The model under review builds one solid part; all positions refer to its coordinate system, in mm. Face numbers are marked on the shaded views. A direction names the side the tool comes from. Round coordinates to 2 decimals unless told otherwise and drop trailing zeros. Write each loop counter-clockwise with the first axis right and the second up, starting at its lowest first coordinate (ties: lowest second). Pieces come first, ordered by that corner, then holes. Notation, with made-up numbers: (28, -16.5) - (84, -16.5) arc R16 ccw to (84, 14.5) - close; hole circle Ø2 at (75, 54). An arc over 180 degrees is marked (long way). Return JSON: item names as keys, results as strings.
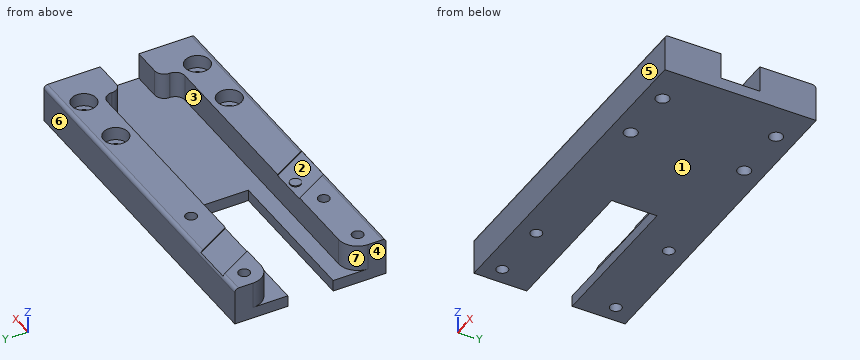
from build123d import *

# Parameters (mm, degrees)
SKETCH_1_W           = 255
SKETCH_1_H           = 80
EXTRUDE_1_DEPTH      = 5
SKETCH_2_R           = 5
CUT_EXTRUDE_1_DEPTH  = 5
SKETCH_3_R           = 4
CUT_EXTRUDE_2_DEPTH  = 10
SKETCH_4_W           = 50
SKETCH_4_H           = 20
EXTRUDE_2_DEPTH      = 10
SKETCH_5_R           = 15
CUT_EXTRUDE_3_DEPTH  = 10
SKETCH_6_R           = 7
EXTRUDE_3_DEPTH      = 15
HOLE_WIZARD_M6_1_D   = 5
CUT_EXTRUDE_4_DEPTH  = 7
HOLE_WIZARD_M4_1_D   = 3.3
FILLET_1_R           = 10
SKETCH_13_R          = 6.969385005
EXTRUDE_5_DEPTH      = 5
SKETCH_14_W          = 5
SKETCH_14_H          = 75
EXTRUDE_6_DEPTH      = 80
SKETCH_15_W          = 20
SKETCH_15_H          = 5
EXTRUDE_7_DEPTH      = 80
EXTRUDE_8_DEPTH      = 5
SKETCH_17_R          = 3
CUT_EXTRUDE_5_DEPTH  = 5
FILLET_2_R           = 1
SKETCH_18_W          = 309.613912266
SKETCH_18_H          = 134.290371586
CUT_EXTRUDE_6_DEPTH  = 81
SKETCH_19_R          = 17
CUT_EXTRUDE_7_DEPTH  = 11
SKETCH_20_W          = 10
SKETCH_20_H          = 10
EXTRUDE_9_DEPTH      = 50
SKETCH_21_R          = 1.75
CUT_EXTRUDE_8_DEPTH  = 11
SKETCH_22_R          = 3.25
CUT_EXTRUDE_9_DEPTH  = 3.5
FILLET_4_R           = 1
EXTRUDE_10_DEPTH     = 40
SKETCH_24_W          = 160
SKETCH_24_H          = 20.5
CUT_EXTRUDE_10_DEPTH = 7
SKETCH_25_W          = 80
SKETCH_25_H          = 12
CUT_EXTRUDE_11_DEPTH = 4
FILLET_5_R           = 5
CUT_EXTRUDE_12_DEPTH = 0.3
SKETCH_27_R          = 1.45
EXTRUDE_11_DEPTH     = 0.3
F_3_0MM_1_D          = 3
FILLET_6_R           = 2.5


with BuildPart() as part:
    # 草图1 → 凸台-拉伸1 (new body)
    with BuildSketch(Plane.XY):
        Rectangle(SKETCH_1_W, SKETCH_1_H)
    extrude(amount=EXTRUDE_1_DEPTH)

    # 草图2 → 切除-拉伸1 (cut)
    with BuildSketch(Plane.XY.offset(5)):
        with Locations((-107.5, 0)):
            Circle(SKETCH_2_R)
    extrude(amount=-CUT_EXTRUDE_1_DEPTH, mode=Mode.SUBTRACT)

    # 草图3 → 切除-拉伸2 (cut)
    with BuildSketch(Plane.XY.offset(5)):
        with Locations((-45, 0)):
            Circle(SKETCH_3_R)
    extrude(amount=-CUT_EXTRUDE_2_DEPTH, mode=Mode.SUBTRACT)

    # 草图4 → 凸台-拉伸2 (add)
    with BuildSketch(Plane.XY.offset(5)):
        with Locations((-22.5, 0)):
            Rectangle(SKETCH_4_W, SKETCH_4_H)
    extrude(amount=EXTRUDE_2_DEPTH)

    # 草图5 → 切除-拉伸3 (cut)
    with BuildSketch(Plane.XY.offset(5)):
        with Locations((70, 0)):
            Circle(SKETCH_5_R)
    extrude(amount=-CUT_EXTRUDE_3_DEPTH, mode=Mode.SUBTRACT)

    # 草图6 → 凸台-拉伸3 (add)
    with BuildSketch(Plane(origin=(0, 0, 0), x_dir=(-1, 0, 0), z_dir=(0, 0, -1))):
        with Locations((107.5, 0)):
            Circle(SKETCH_6_R)
    extrude(amount=-EXTRUDE_3_DEPTH)

    # M6 螺纹孔1 (through all)
    with Locations(Plane.XY.offset(15)):
        with Locations((-107.5, 0)):
            Hole(HOLE_WIZARD_M6_1_D / 2)

    # 草图10 → 切除-拉伸4 (cut)
    with BuildSketch(Plane.XY.offset(15)):
        with BuildLine():
            Line((-47.5, 5.1), (2.5, 5.1))
            ThreePointArc((2.5, 5.1), (7.6, 0), (2.5, -5.1))
            Line((2.5, -5.1), (-47.5, -5.1))
            ThreePointArc((-47.5, -5.1), (-52.6, 0), (-47.5, 5.1))
        make_face()
    extrude(amount=-CUT_EXTRUDE_4_DEPTH, mode=Mode.SUBTRACT)

    # M4 螺纹孔1 (through all)
    with Locations(Plane(origin=(0, 0, 0), x_dir=(-1, 0, 0), z_dir=(0, 0, -1))):
        with Locations((-39.75, -26.5), (-39.75, -1.5), (-109.94007449, -26.5), (-100.25, -1.5)):
            Hole(HOLE_WIZARD_M4_1_D / 2)

    # 圆角1
    fillet_1_edges = [part.edges().sort_by_distance(p)[0] for p in [
        (-127.5, 40, 2.5),
        (-127.5, -40, 2.5),
    ]]
    fillet(fillet_1_edges, radius=FILLET_1_R)

    # 草图13 → 凸台-拉伸5 (add)
    with BuildSketch(Plane.XY.offset(5)):
        with Locations((-45, 0)):
            Circle(SKETCH_13_R)
    extrude(amount=-EXTRUDE_5_DEPTH)

    # 草图14 → 凸台-拉伸6 (add)
    with BuildSketch(Plane.XZ.offset(40)):
        with Locations((125, -37.5)):
            Rectangle(SKETCH_14_W, SKETCH_14_H)
    extrude(amount=-EXTRUDE_6_DEPTH)

    # 草图15 → 凸台-拉伸7 (add)
    with BuildSketch(Plane.XZ.offset(40)):
        with Locations((112.5, -72.5)):
            Rectangle(SKETCH_15_W, SKETCH_15_H)
    extrude(amount=-EXTRUDE_7_DEPTH)

    # 草图16 → 凸台-拉伸8 (add)
    with BuildSketch(Plane.XZ.offset(40)):
        Polygon((-32.5, 5), (-32.5, 0), (102.5, -75), (127.5, -75), (127.5, 5), align=None)
    extrude_8 = extrude(amount=-EXTRUDE_8_DEPTH)

    # 镜向1: 凸台-拉伸8 across plane
    add(extrude_8.mirror(Plane.ZX))

    # 草图17 → 切除-拉伸5 (cut)
    with BuildSketch(Plane(origin=(0, 0, -75), x_dir=(-1, 0, 0), z_dir=(0, 0, -1))):
        with Locations((-114.5, -15)):
            Circle(SKETCH_17_R)
        with Locations((-114.5, 15)):
            Circle(SKETCH_17_R)
    extrude(amount=-CUT_EXTRUDE_5_DEPTH, mode=Mode.SUBTRACT)

    # 圆角2
    fillet_2_edges = [part.edges().sort_by_distance(p)[0] for p in [
        (-75, -40, 0),
        (5, -40, 5),
        (-127.5, 0, 0),
        (-124.571067812, 37.071067812, 0),
        (-124.571067812, -37.071067812, 0),
        (-127.5, 0, 5),
        (-124.571067812, 37.071067812, 5),
        (-124.571067812, -37.071067812, 5),
        (127.5, 0, 5),
        (127.5, 0, -75),
        (115, -40, -75),
        (115, 40, -75),
        (35, -40, -37.5),
        (35, -35, -37.5),
        (5, 40, 5),
        (-75, 40, 0),
        (35, 40, -37.5),
        (35, 35, -37.5),
        (127.5, 40, -35),
        (127.5, -40, -35),
    ]]
    fillet(fillet_2_edges, radius=FILLET_2_R)

    # 草图18 → 切除-拉伸6 (cut, through all)
    with BuildSketch(Plane.XY.offset(5)):
        Rectangle(SKETCH_18_W, SKETCH_18_H)
    extrude(amount=-CUT_EXTRUDE_6_DEPTH, mode=Mode.SUBTRACT)

    # 草图19 → 切除-拉伸7 (cut, through all)
    with BuildSketch(Plane.XY.offset(15)):
        with Locations((-107.5, 0)):
            Circle(SKETCH_19_R)
    extrude(amount=-CUT_EXTRUDE_7_DEPTH, mode=Mode.SUBTRACT)

    # 草图20 → 凸台-拉伸9 (add)
    with BuildSketch(Plane(origin=(2.5, 0, 0), x_dir=(0, 0, -1), z_dir=(1, 0, 0))):
        with Locations((-10, 15)):
            Rectangle(SKETCH_20_W, SKETCH_20_H)
    extrude_9 = extrude(amount=-EXTRUDE_9_DEPTH)

    # 镜向2: 凸台-拉伸9 across plane
    add(extrude_9.mirror(Plane.ZX))

    # 草图21 → 切除-拉伸8 (cut, through all)
    with BuildSketch(Plane.XY.offset(15)):
        with Locations((-22.5, 15)):
            Circle(SKETCH_21_R)
        with Locations((-7.5, 15)):
            Circle(SKETCH_21_R)
        with Locations((-7.5, -15)):
            Circle(SKETCH_21_R)
        with Locations((-22.5, -15)):
            Circle(SKETCH_21_R)
    extrude(amount=-CUT_EXTRUDE_8_DEPTH, mode=Mode.SUBTRACT)

    # 草图22 → 切除-拉伸9 (cut)
    with BuildSketch(Plane.XY.offset(15)):
        with Locations((-22.5, 15)):
            Circle(SKETCH_22_R)
        with Locations((-7.5, 15)):
            Circle(SKETCH_22_R)
        with Locations((-7.5, -15)):
            Circle(SKETCH_22_R)
        with Locations((-22.5, -15)):
            Circle(SKETCH_22_R)
    extrude(amount=-CUT_EXTRUDE_9_DEPTH, mode=Mode.SUBTRACT)

    # 圆角4
    fillet_4_edges = [part.edges().sort_by_distance(p)[0] for p in [
        (-22.5, 20, 15),
        (-22.5, -20, 15),
    ]]
    fillet(fillet_4_edges, radius=FILLET_4_R)

    # 草图23 → 凸台-拉伸10 (add)
    with BuildSketch(Plane.ZY.offset(47.5)):
        with BuildLine():
            Line((5, -20), (14, -20))
            ThreePointArc((14, -20), (14.707106781, -19.707106781), (15, -19))
            Line((15, -19), (15, -5.1))
            Line((15, -5.1), (8, -5.1))
            Line((8, -5.1), (8, 5.1))
            Line((8, 5.1), (15, 5.1))
            Line((15, 5.1), (15, 19))
            ThreePointArc((15, 19), (14.707106781, 19.707106781), (14, 20))
            Line((14, 20), (5, 20))
            Line((5, 20), (5, -20))
        make_face()
    extrude(amount=EXTRUDE_10_DEPTH)

    # 草图24 → 切除-拉伸10 (cut)
    with BuildSketch(Plane.XY.offset(15)):
        with Locations((-87.5, 0)):
            Rectangle(SKETCH_24_W, SKETCH_24_H)
    extrude(amount=-CUT_EXTRUDE_10_DEPTH, mode=Mode.SUBTRACT)

    # 草图25 → 切除-拉伸11 (cut, through all)
    with BuildSketch(Plane.XY.offset(8)):
        with Locations((-87.5, 0)):
            Rectangle(SKETCH_25_W, SKETCH_25_H)
    extrude(amount=-CUT_EXTRUDE_11_DEPTH, mode=Mode.SUBTRACT)

    # 圆角5
    fillet_5_edges = [part.edges().sort_by_distance(p)[0] for p in [
        (-87.5, 10.25, 11.5),
        (-87.5, -10.25, 11.5),
    ]]
    fillet(fillet_5_edges, radius=FILLET_5_R)

    # 草图26 → 切除-拉伸12 (cut)
    with BuildSketch(Plane.XY.offset(15)):
        Polygon((-58.521459286, -20), (-81.615470054, 20), (-71.223165208, 20), (-48.129154441, -20), align=None)
    extrude(amount=-CUT_EXTRUDE_12_DEPTH, mode=Mode.SUBTRACT)

    # 草图27 → 凸台-拉伸11 (add)
    with BuildSketch(Plane.XY.offset(14.7)):
        with Locations((-58.285898385, -12.408003449)):
            Circle(SKETCH_27_R)
    extrude(amount=EXTRUDE_11_DEPTH)

    # Ø3.0mm 暗销孔1 (through all)
    with Locations(Plane.XY.offset(15)):
        with Locations((-83, 15), (-58, 15), (-67, -15), (-83, -15)):
            Hole(F_3_0MM_1_D / 2)

    # 圆角6
    fillet_6_edges = [part.edges().sort_by_distance(p)[0] for p in [
        (-7.5, -5.1, 11.5),
        (-7.5, 5.1, 11.5),
        (-7.5, 10.25, 11.5),
        (-7.5, -10.25, 11.5),
    ]]
    fillet(fillet_6_edges, radius=FILLET_6_R)


solid = part.part
(1) Add section A-A (x = -22.5). Write out the cut boundary in (y, z).
Filled in:
{"outline": "(-20, 5) - (-16.75, 5) - (-16.75, 11.5) - (-18.25, 11.5) - (-18.25, 15) - (-19, 15) arc R1 ccw to (-20, 14) - close; (-13.25, 5) - (13.25, 5) - (13.25, 11.5) - (11.75, 11.5) - (11.75, 15) - (10.25, 15) - (10.25, 8) - (-10.25, 8) - (-10.25, 15) - (-11.75, 15) - (-11.75, 11.5) - (-13.25, 11.5) - close; (16.75, 5) - (20, 5) - (20, 14) arc R1 ccw to (19, 15) - (18.25, 15) - (18.25, 11.5) - (16.75, 11.5) - close"}
(2) Wall thickness on line 1 (Y direction, x = -67, z = 11.5); line 2 (Y direction, x = -58, z = 12.5); line 3 (Y direction, x = -83, z = 7): over which ranges is each line inside the solid? List them lowest first.
Filled in:
{"line 1": "y = -20 to -16.5, -13.5 to -10.25, 10.25 to 20", "line 2": "y = -20 to -10.25, 10.25 to 13.5, 16.5 to 20", "line 3": "y = -20 to -16.5, -13.5 to -6, 6 to 13.5, 16.5 to 20"}
(3) Mouldability with a two-part tool opening along Y and no side actions: class the marked faces 4, 5, 6 and 7 as released by +Y, released by -Y, zero draft, split by the parting line, or undercut.
Filled in:
{"face 4": "zero draft", "face 5": "released by -Y", "face 6": "released by +Y", "face 7": "undercut"}
(4) For the marked faces 1, 2 and 3, list the 3-axis set-ups (+Z, -Z, +X, -X, +Y, -Y) from which the entire face can be reached by the end or side of a thin tool; tool diameter is ignored.
Filled in:
{"face 1": "-Z, +X, -X, +Y, -Y", "face 2": "+Z", "face 3": "+Z, -X"}
(5) Add section C-C (x = -45). Write out the cut boundary in (y, z).
Filled in:
{"outline": "(-20, 5) - (20, 5) - (20, 14) arc R1 ccw to (19, 15) - (10.25, 15) - (10.25, 8) - (-10.25, 8) - (-10.25, 15) - (-19, 15) arc R1 ccw to (-20, 14) - close"}
(6) Clearance check with flat-ended pins moving along their axes: pin 1 Ø5 at (x, y) = (-22.5, 15) entering from +Z; pin 2 Ø7 at (x, y) = (-6.5, 15) entering from +Z; pin 3 Ø1.5 at (x, y) = (-53.5, 5) entering from +Z; pin 4 Ø1.5 at (y, z) = (-0.5, 7) entering from -X. State where each tip first meets the part, or that it passes through.
Filled in:
{"pin 1": "stops at z = 11.5", "pin 2": "stops at z = 15", "pin 3": "passes through", "pin 4": "stops at x = -47.5"}
(7) Add section B-B (x = -61.5). Write out the cut boundary in (y, z).
Filled in:
{"outline": "(-20, 5) - (-6, 5) - (-6, 8) - (-10.25, 8) - (-10.25, 14.7) - (-14.84, 14.7) - (-14.84, 15) - (-19, 15) arc R1 ccw to (-20, 14) - close; (6, 5) - (20, 5) - (20, 14) arc R1 ccw to (19, 15) - (10.25, 15) - (10.25, 8) - (6, 8) - close"}
